from build123d import *

# Parameters (mm, degrees)
SKETCH1_R           = 12
SKETCH1_R_2         = 3.5
BOSS_EXTRUDE1_DEPTH = 0.5
SKETCH2_W           = 14
SKETCH2_H           = 6
BOSS_EXTRUDE2_DEPTH = 5
SKETCH3_W           = 13
SKETCH3_H           = 4
CUT_EXTRUDE1_DEPTH  = 5
SKETCH4_W           = 8
SKETCH4_H           = 5
CUT_EXTRUDE2_DEPTH  = 4.5
BOSS_EXTRUDE3_DEPTH = 5


with BuildPart() as part:
    # Sketch1 → Boss-Extrude1 (new body, symmetric)
    with BuildSketch(Plane(origin=(0, 0, 0), x_dir=(1, 0, 0), z_dir=(0, 1, 0))):
        Circle(SKETCH1_R)
        Circle(SKETCH1_R_2, mode=Mode.SUBTRACT)
    extrude(amount=BOSS_EXTRUDE1_DEPTH, both=True)

    # Sketch2 → Boss-Extrude2 (add)
    with BuildSketch(Plane(origin=(0, 0.5, 0), x_dir=(1, 0, 0), z_dir=(0, 1, 0))):
        with Locations((0, 11)):
            Rectangle(SKETCH2_W, SKETCH2_H)
    extrude(amount=BOSS_EXTRUDE2_DEPTH)

    # Sketch3 → Cut-Extrude1 (cut)
    with BuildSketch(Plane(origin=(0, 0, -14), x_dir=(-1, 0, 0), z_dir=(0, 0, -1))):
        with Locations((0, 3)):
            Rectangle(SKETCH3_W, SKETCH3_H)
    extrude(amount=-CUT_EXTRUDE1_DEPTH, mode=Mode.SUBTRACT)

    # Sketch4 → Cut-Extrude2 (cut)
    with BuildSketch(Plane(origin=(0, 5.5, 0), x_dir=(1, 0, 0), z_dir=(0, 1, 0))):
        with Locations((0, 11.5)):
            Rectangle(SKETCH4_W, SKETCH4_H)
    extrude(amount=-CUT_EXTRUDE2_DEPTH, mode=Mode.SUBTRACT)

    # Sketch5 → Boss-Extrude3 (add)
    with BuildSketch(Plane(origin=(0, 0.5, 0), x_dir=(1, 0, 0), z_dir=(0, 1, 0))):
        Polygon((-6.491303756, -4.950065272), (-2.866072607, -6.640538319), (-3.5, -8), (-7.125231148, -6.309526953), align=None)
        Polygon((7.125231148, -6.309526953), (6.491303756, -4.950065272), (2.866072607, -6.640538319), (3.5, -8), align=None)
    extrude(amount=BOSS_EXTRUDE3_DEPTH)


solid = part.part
The listing builds one solid part. Answer for the finished solid, in the listing's coordinates (mm). A direction names the side the tool comes from. Coordinates: 2 decimals unless noted, no trailing zeros. Loops run counter-clockwise (first coordinate to the right, second up) from the corner with the lowest first, then second, coordinate; pieces in that order, holes last.
1) Determine the mould class of faces 5 (the face through (4.704, 2.965, 5.783)), 6 (the face through (6.5, 3, -12)), 7 (the face through (6.813, 2.965, 5.639)), 8 (the face through (0, 3, -8)) for opening direction X: pulls with the +X half, pulls with the -X half, needs draft (parallel to the pull), parting line crosses it, or undercut.
2) Find section B-B on z = 0. Write down the section's boundary in (x, y).
3) A tool of negligible diameter and unlimited length cuts with its end or side. For faces 1 (the face through (-7, 3, -11)), 2 (the face through (3.18, 2.96, 7.31)), 3 (the face through (5, 5, -12)), 4 (the face through (5.287, 2.965, 7.167)), from which of +Z, -Z, +X, -X, +Y, -Y can it reach the whole face along a straight path? Write none if from no direction.
4) Flat-ended cylindrical pins translate along their axes: pin 1 Ø2 at (x, y) = (1, 3.5) entering from -Z; pin 2 Ø1.5 at (x, z) = (-8.5, 8.5) entering from +Y; pin 3 Ø2 at (y, z) = (3.5, -12) entering from -X; pin 4 Ø1 at (x, y) = (-9, 4.5) entering from +Z. Find the tip coordinate at first contact, or state that the pin passes through.
5) Find section A-A on y = 2.5. Write down the section's boundary in (x, z).
6) Find section D-D on z = -12.5. Write down the section's boundary in (x, y), then the cut area to 3 significant figures.
7) Find section C-C on x = 0. Write down the section's boundary in (y, z).
8) Find the intervals of material crossed by L1, parallel to Z at x = 0, y = 0.2; L2, parallel to Z at x = 1.75, y = 0.8, in increasing order.
Values:
1. face 5: undercut
1. face 6: undercut
1. face 7: pulls with the +X half
1. face 8: needs draft
2. outline: (-12, -0.5) - (-3.5, -0.5) - (-3.5, 0.5) - (-12, 0.5) - close; (3.5, -0.5) - (12, -0.5) - (12, 0.5) - (3.5, 0.5) - close
3. face 1: -Z, -X, +Y
3. face 2: +Z, +Y
3. face 3: -Z
3. face 4: +Z, +X, +Y
4. pin 1: stops at z = -9
4. pin 2: stops at y = 0.5
4. pin 3: stops at x = -7
4. pin 4: passes through
5. outline: (-7.13, 6.31) - (-6.49, 4.95) - (-2.87, 6.64) - (-3.5, 8) - close; (-7, -14) - (-6.5, -14) - (-6.5, -9) - (6.5, -9) - (6.5, -14) - (7, -14) - (7, -8) - (-7, -8) - close; (2.87, 6.64) - (6.49, 4.95) - (7.13, 6.31) - (3.5, 8) - close
6. outline: (-7, 0.5) - (7, 0.5) - (7, 5.5) - (4, 5.5) - (4, 5) - (6.5, 5) - (6.5, 1) - (-6.5, 1) - (-6.5, 5) - (-4, 5) - (-4, 5.5) - (-7, 5.5) - close
6. area: 14.0 mm2
7. outline: (-0.5, -12) - (0.5, -12) - (0.5, -14) - (1, -14) - (1, -9) - (5.5, -9) - (5.5, -8) - (0.5, -8) - (0.5, -3.5) - (-0.5, -3.5) - close; (-0.5, 3.5) - (0.5, 3.5) - (0.5, 12) - (-0.5, 12) - close
8. L1: z = -12 to -3.5, 3.5 to 12
8. L2: z = -14 to -8
